```python
from build123d import *

# Parameters (mm, degrees)
F2_T      = -0.75
F4_D      = 2
F4_DEPTH  = 2.751
F6_D      = 2
F8_D      = 2
F8_DEPTH  = 2.751
F10_D     = 2
F12_D     = 2
F12_DEPTH = 2.751
F14_D     = 2


with BuildPart() as f1:
    # F0 (on Top) → F1 (revolve)
    with BuildSketch(Plane.XY):
        with BuildLine():
            ThreePointArc((2.75, 0), (0, 2.75), (-2.75, 0))
            Line((-2.75, 0), (2.75, 0))
        make_face()
    revolve(axis=Axis((0.1047021379, 0, 0), (1, 0, 0)))

    # F2 (hollow: no face is removed)
    offset(amount=F2_T, mode=Mode.SUBTRACT)

    # F4 (through all, one way)
    with BuildSketch(Plane.XY):
        with Locations((0, 0)):
            Circle(F4_D / 2)
    extrude(amount=-F4_DEPTH, mode=Mode.SUBTRACT)

    # F6 (through all)
    with Locations(Plane(origin=(0, 0, 0), x_dir=(1, 0, 0), z_dir=(0, 0, -1))):
        with Locations((0, 0)):
            Hole(F6_D / 2)

    # F8 (through all, one way)
    with BuildSketch(Plane.YZ):
        with Locations((0, 0)):
            Circle(F8_D / 2)
    extrude(amount=-F8_DEPTH, mode=Mode.SUBTRACT)

    # F10 (through all)
    with Locations(Plane(origin=(0, 0, 0), x_dir=(0, 1, 0), z_dir=(-1, 0, 0))):
        with Locations((0, 0)):
            Hole(F10_D / 2)

    # F12 (through all, one way)
    with BuildSketch(Plane.XZ):
        with Locations((0, 0)):
            Circle(F12_D / 2)
    extrude(amount=-F12_DEPTH, mode=Mode.SUBTRACT)

    # F14 (through all)
    with Locations(Plane(origin=(0, 0, 0), x_dir=(1, 0, 0), z_dir=(0, 1, 0))):
        with Locations((0, 0)):
            Hole(F14_D / 2)


solid = f1.part
```
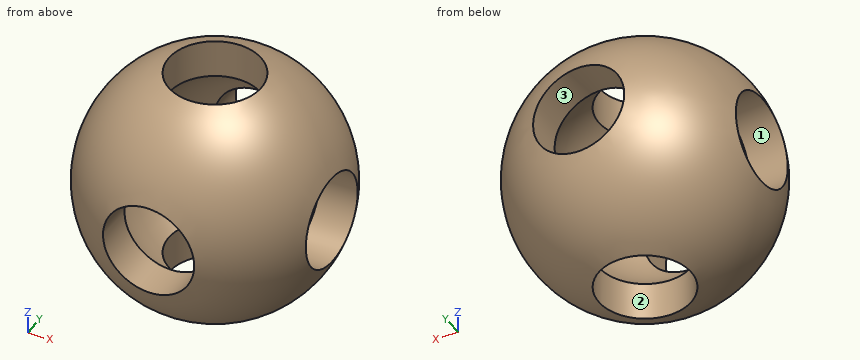
The listing builds one solid part. Answer for the finished solid, in the listing's coordinates (mm). Face numbers are marked on the shaded views. Coordinates: 2 decimals unless noted, no trailing zeros. Write each loop counter-clockwise with the first axis right and the second up, starting at its lowest first coordinate (ties: lowest second). Pieces come first, ordered by that corner, then holes. Notation, with made-up numbers: (70, 84) - (88, 84) arc R13 cw to (88, 90) - close; hole circle Ø3 at (21.5, 4.5). An arc over 180 degrees is marked (long way). Return JSON: item names as keys, results as strings. Group by question number.
Q1. Find the intervals of material crossed by line 1 along Z through (x, y) = (2.2, 0); line 2 along X through (y, z) = (-0.95, -1.2); line 3 along Y through (x, z) = (-0.1, 2.05), in increasing order. Write a range as [from, to].
Q2. The part is cut by section D-D on z = 1.5. Write down the section's boundary in (x, y).
Q3. For a pull along Y with two mould halves and no side action, classify the marked faces 1, 2 and 3 as +Y half, -Y half, draft (parallel to the pull), parting line (faces both ways), or undercut.
Q4. Flat-ended cylindrical pins translate along their axes: pin 1 Ø1.2 at (y, z) = (0, 0) entering from +X; pin 2 Ø1 at (x, y) = (0.5, 1.5) entering from -Z; pin 3 Ø2.5 at (x, y) = (0, 0) entering from +Z; pin 4 Ø1 at (x, y) = (1.5, -1.5) entering from +Z. Find the tip coordinate at first contact, or state that the pin passes through.
Q5. The part is cut by section A-A on x = 0. Write down the section's boundary in (y, z), and give its area (3 significant figures).
Q6. The part is cut by section C-C on y = -1.9. Write down the section's boundary in (x, z).
Evaluation:
{
 "1": {"line 1": "z = [-1.65, -1], [1, 1.65]", "line 2": "x = [-2.28, -1.29], [1.29, 2.28]", "line 3": "y = [-1.83, -0.99], [0.99, 1.83]"},
 "2": {"outline": "circle Ø4.61 at (0, 0); hole circle Ø2.65 at (0, 0)"},
 "3": {"face 1": "undercut", "face 2": "undercut", "face 3": "draft"},
 "4": {"pin 1": "passes through", "pin 2": "stops at z = -2.53", "pin 3": "stops at z = 2.56", "pin 4": "stops at z = 2.22"},
 "5": {"outline": "(-2.56, -1) arc R2.75 ccw to (-1, -2.56) - (-1, -1.73) arc R2 cw to (-1.73, -1) - close; (-2.56, 1) - (-1.73, 1) arc R2 cw to (-1, 1.73) - (-1, 2.56) arc R2.75 ccw to start; (1, -2.56) arc R2.75 ccw to (2.56, -1) - (1.73, -1) arc R2 cw to (1, -1.73) - close; (1, 1.73) arc R2 cw to (1.73, 1) - (2.56, 1) arc R2.75 ccw to (1, 2.56) - close", "area": "4.99 mm2"},
 "6": {"outline": "circle Ø3.98 at (0, 0); hole circle Ø2 at (0, 0)"}
}
